```python
from build123d import *

# Parameters (mm, degrees)
F0_R     = 7.5
F1_DEPTH = 20


with BuildPart() as f1:
    # F0 (on Top) → F1 (new body)
    with BuildSketch(Plane.XY):
        Polygon((218, 380), (218, 584), (-218, 584), (-218, 380), (-328.044827, 189.396769), (-438.089653, -1.206462), (-614.758836, -103.206462), (-396.758836, -480.793538), (-220.089653, -378.793538), (0, -378.793538), (220.089653, -378.793538), (396.758836, -480.793538), (614.758836, -103.206462), (438.089653, -1.206462), (328.044827, 189.396769), align=None)
        with Locations((-484.108201, -279.5)):
            Circle(F0_R, mode=Mode.SUBTRACT)
        Polygon((-372.271723, 36.793538), (-323.19695, 121.793538), (-56.122177, -340.793538), (-154.271723, -340.793538), align=None, mode=Mode.SUBTRACT)
        with Locations((484.108201, -279.5)):
            Circle(F0_R, mode=Mode.SUBTRACT)
        Polygon((154.271723, -340.793538), (56.122177, -340.793538), (323.19695, 121.793538), (372.271723, 36.793538), align=None, mode=Mode.SUBTRACT)
        Polygon((-295.135861, 170.396769), (-284.395281, 189), (0, 189), (284.395281, 189), (295.135861, 170.396769), (305.876442, 151.793538), (163.678801, -94.5), (21.481161, -340.793538), (0, -340.793538), (-21.481161, -340.793538), (-163.678801, -94.5), (-305.876442, 151.793538), align=None, mode=Mode.SUBTRACT)
        Polygon((-218, 304), (218, 304), (267.074773, 219), (-267.074773, 219), align=None, mode=Mode.SUBTRACT)
        with Locations((0, 559)):
            Circle(F0_R, mode=Mode.SUBTRACT)
    extrude(amount=F1_DEPTH)


solid = f1.part
```
For this review, take the finished solid that the model builds, in its own axes (mm). A direction names the side the tool comes from. Round coordinates to 2 decimals unless told otherwise and drop trailing zeros. Write each loop counter-clockwise with the first axis right and the second up, starting at its lowest first coordinate (ties: lowest second). Pieces come first, ordered by that corner, then holes. Notation, with made-up numbers: (13.25, 74) - (35.25, 74) arc R31 ccw to (35.25, 104) - close; hole circle Ø9 at (87, -14). An arc over 180 degrees is marked (long way). Put each result on its own line as item: value.
Q1. We need section B-B (x = 358). Give the boundary of the cut face in (y, z).
Solved:
outline: (-458.42, 0) - (12.07, 0) - (12.07, 20) - (-458.42, 20) - close; (61.51, 0) - (137.51, 0) - (137.51, 20) - (61.51, 20) - close
Q2. We need section D-D (y = 396.5). Give the boundary of the cut face in (x, z).
Solved:
outline: (-218, 0) - (218, 0) - (218, 20) - (-218, 20) - close
Q3. We need section C-C (z = 12.5). Count the separate pieces of the cut face and the enclosed holes in it, and give its area (3 significant figures).
Solved:
separate pieces: 1
enclosed holes: 7
area: 458,000 mm2
Q4. Mouldability with a two-part tool opening along X and no side actions: class faces 1 (the face through (179, -104, 20)), 2 (the face through (-507.285, -289.357, 9.86)), 3 (the face through (-191.53, -106.26, 9.86)) as released by +X, released by -X, zero draft, split by the parting line, or undercut.
Solved:
face 1: zero draft
face 2: released by -X
face 3: undercut
Q5. Insertion check: pin 1 Ø6 at (x, z) = (-75, 12.5) entering from -Y; pin 2 Ø10 at (x, z) = (388, 2.5) entering from +Y; pin 3 Ø2 at (y, z) = (198.5, 7.5) entering from -X. Each pin has a flat end and moves straight along its axis. Give the tip position at first contact, or say it passes through.
Solved:
pin 1: stops at y = -378.79
pin 2: stops at y = 94.21
pin 3: stops at x = -323.37
Q6. Wall thickness on probe 1 along X at (y, z) = (-312, 16.25); probe 2 along Y at (x, z) = (-1.5, 14.5); probe 3 along X at (y, z) = (-279.5, 5.5): over which ranges is each line inside the solid? List them lowest first.
Solved:
probe 1: x = -494.21 to -170.9, -72.75 to -38.11, 38.11 to 72.75, 170.9 to 494.21
probe 2: y = -378.79 to -340.79, 189 to 219, 304 to 551.65, 566.35 to 584
probe 3: x = -512.98 to -491.61, -476.61 to -189.66, -91.51 to -56.87, 56.87 to 91.51, 189.66 to 476.61, 491.61 to 512.98
Q7. Machinability: for faces 4 (the face through (179, -104, 0)), 5 (the face through (-348.078, 78.699, 9.86)), 6 (the face through (-309.661, -430.508, 9.86)), which of the approach directions +Z, -Z, +X, -X, +Y, -Y give a long, thin tool a straight path to every point of the face, cutting with its end or side? Answer none if there is none.
Solved:
face 4: -Z, +X, -X, +Y, -Y
face 5: +Z, -Z
face 6: +Z, -Z, -Y
Q8. We need section A-A (y = -24.5). Give the boundary of the cut face in (x, z), and give its area (3 significant figures).
Solved:
outline: (-478.44, 0) - (-336.88, 0) - (-336.88, 20) - (-478.44, 20) - close; (-238.73, 0) - (-204.09, 0) - (-204.09, 20) - (-238.73, 20) - close; (204.09, 0) - (238.73, 0) - (238.73, 20) - (204.09, 20) - close; (336.88, 0) - (478.44, 0) - (478.44, 20) - (336.88, 20) - close
area: 7,050 mm2
